Check sheet for the modelled part. Datum: model origin and axes. Units: mm. A direction names the side the tool comes from. Give positions to 0.01 mm unless a question says otherwise; leave off trailing zeros. Order: outer loops, then holes, each group sorted by start corner. A loop starts at its lowest first (then second) coordinate and runs counter-clockwise, first axis right, second up.
Autodesk Fusion 360 part; units mm, degrees
sketch "Skizze1" plane through (0, 0, 0) normal (0, 0, 1) x (1, 0, 0)
  line L0 (15.25, -4.5) -> (-15.25, -4.5)
  line L1 (-15.25, -4.5) -> (-15.25, 4.5)
  line L2 (-15.25, 4.5) -> (15.25, 4.5)
  line L3 (15.25, 4.5) -> (15.25, -4.5)
  line L4 (15.25, -4.5) -> (-15.25, 4.5) construction
  line L5 (-15.25, -4.5) -> (15.25, 4.5) construction
  line L6 (17.25, -6.5) -> (-17.25, -6.5)
  line L7 (-17.25, -6.5) -> (-17.25, 6.5)
  line L8 (-17.25, 6.5) -> (17.25, 6.5)
  line L9 (17.25, 6.5) -> (17.25, -6.5)
  line L10 (17.25, -6.5) -> (-17.25, 6.5) construction
  line L11 (-17.25, -6.5) -> (17.25, 6.5) construction
  dimension "d1" = 30.5
  dimension "d2" = 9
  dimension "d3" = 34.5
  dimension "d4" = 13
extrude "Extrusion1" add sketch "Skizze1" against normal blind 2 contours L0 L1 L2 L3 | L6 L7 L8 L9
extrude "Extrusion2" add sketch "Skizze1" along normal blind 58
fillet "Abrundung1" radius 2 4 edges at (-17.25, -6.5, 28) (-17.25, 6.5, 28) (17.25, -6.5, 28) (17.25, 6.5, 28)
sketch "Skizze2" plane through (0, -6.5, 0) normal (0, -1, 0) x (1, 0, 0)
  line L0 (15.25, -2) -> (15.25, 58)
  line L1 (15.25, 58) -> (-15.25, 58)
  line L2 (-15.25, 58) -> (-15.25, -2)
  line L3 (-15.25, -2) -> (15.25, -2)
  line L4 (-6.75, 3) -> (-0.75, 3)
  line L5 (-0.75, 3) -> (-0.75, 29)
  line L6 (-0.75, 29) -> (-6.75, 29)
  line L7 (-6.75, 29) -> (-6.75, 3)
  line L8 (-17.25, 58) -> (-17.25, -2)
  line L9 (17.25, 0) -> (-17.25, 0)
  dimension "d11" = 6
  dimension "d12" = 26
  dimension "d19" = 8.5
  dimension "d20" = 3
extrude "Extrusion3" cut sketch "Skizze2" against normal blind 2 contours L4 L5 L6 L7
fillet "Abrundung2" radius 2 4 edges at (-0.75, -5.5, 29) (-6.75, -5.5, 29) (-0.75, -5.5, 3) (-6.75, -5.5, 3)
sketch "Skizze3" plane through (0, 6.5, 0) normal (0, 1, 0) x (-1, 0, 0)
  line L0 (-15.25, 58) -> (-15.25, -2)
  line L1 (-15.25, -2) -> (15.25, -2)
  line L2 (15.25, -2) -> (15.25, 58)
  line L3 (15.25, 58) -> (-15.25, 58)
  line L4 (-12.25, 50) -> (5.75, 50)
  line L5 (6.75, 49) -> (6.75, 48)
  line L6 (5.75, 47) -> (-12.25, 47)
  line L7 (-13.25, 48) -> (-13.25, 49)
  line L8 (-15.25, 0) -> (15.25, 0)
  arc A0 (-12.25, 50) -> (-13.25, 49) centre (-12.25, 49) ccw
  arc A1 (-13.25, 48) -> (-12.25, 47) centre (-12.25, 48) ccw
  arc A2 (5.75, 47) -> (6.75, 48) centre (5.75, 48) ccw
  arc A3 (6.75, 49) -> (5.75, 50) centre (5.75, 49) ccw
  point P0 (-13.25, 50)
  point P1 (6.75, 50)
  dimension "d21" = 47
  dimension "d22" = 50
  dimension "d23" = 20
  dimension "d24" = 2
  dimension "d27" = 1
extrude "Extrusion4" cut sketch "Skizze3" against normal blind 3 contours L4 L5 L6 L7 A0 A1 A2 A3
equation "d3 = d1 + ( ( 2 * 2 ) * 1 mm )"
equation "d4 = d2 + ( ( 2 * 2 ) * 1 mm )"
equation "d12 = 28 mm - 2 mm"
Q1. Draft check along X on faces 6 (the cylindrical face through (-6.15, -5.49, 3.57)), 7 (the flat face through (-17.25, 0, 28)), 8 (the cylindrical face through (16.65, -5.93, 28.42)). Enter one of: pulls with the +X half, pulls with the -X half, needs draft (parallel to the pull), parting line crosses it, or undercut.
Q2. Sectioned sample at D-D, the plane y = 3.75. Record the cut outline in (x, z).
Q3. Sectioned sample at A-A, the plane y = -5.5. Record the cut outline in (x, z), plus the area to 3 significant figures.
Q4. Go/stop test with a flat-tipped pin: P1, Ø1, axis at y = -5.5, z = 21.5, coming from the +X side. Record where the tip stops, or that it passes through.
Q5. Tool access check on faces 1 (the flat face through (17.25, 0, 28)), 2 (the flat face through (3, 6, 47)), 3 (the cylindrical face through (-1.35, -5.49, 28.43)), 4 (the cylindrical face through (16.68, 5.9, 28.42)), 5 (the flat face through (-15.25, 0, 29)). Record the directions out of +Z, -Z, +X, -X, +Y, -Y that give a thin tool (end or side, any length) a straight path to the whole face; none if there is none.
Q6. Sectioned sample at C-C, the plane z = 36. Record the cut outline in (x, y).
Q7. Sectioned sample at B-B, the plane x = -14. Record the cut outline in (y, z).
Q8. Material ranges on line 1 (Y direction, x = -11, z = 32); line 2 (X direction, y = -1, z = 19); line 3 (Z direction, x = 0, y = -0.5), recorded low to high.
Filled in:
1. face 6: undercut
1. face 7: pulls with the -X half
1. face 8: pulls with the +X half
2. outline: (-17.25, -2) - (17.25, -2) - (17.25, 58) - (15.25, 58) - (15.25, 0) - (-15.25, 0) - (-15.25, 58) - (-17.25, 58) - close
3. outline: (-16.98, -2) - (16.98, -2) - (16.98, 58) - (-16.98, 58) - close; hole (-6.75, 5) arc R2 ccw to (-4.75, 3) - (-2.75, 3) arc R2 ccw to (-0.75, 5) - (-0.75, 27) arc R2 ccw to (-2.75, 29) - (-4.75, 29) arc R2 ccw to (-6.75, 27) - close
3. area: 1,890 mm2
4. P1: stops at x = 17.19
5. face 1: +Z, -Z, +X, +Y, -Y
5. face 2: +Y
5. face 3: -Y
5. face 4: +Z, -Z, +X, +Y
5. face 5: +Z
6. outline: (-17.25, -4.5) arc R2 ccw to (-15.25, -6.5) - (15.25, -6.5) arc R2 ccw to (17.25, -4.5) - (17.25, 4.5) arc R2 ccw to (15.25, 6.5) - (-15.25, 6.5) arc R2 ccw to (-17.25, 4.5) - close; hole (-15.25, -4.5) - (15.25, -4.5) - (15.25, 4.5) - (-15.25, 4.5) - close
7. outline: (-6.5, -2) - (6.5, -2) - (6.5, 58) - (4.5, 58) - (4.5, 0) - (-4.5, 0) - (-4.5, 58) - (-6.5, 58) - close
8. line 1: y = -6.5 to -4.5, 4.5 to 6.5
8. line 2: x = -17.25 to -15.25, 15.25 to 17.25
8. line 3: z = -2 to 0
